Can you work these out from the drawing? Everything is in mm from the part's minimum corner. Round coordinates to 2 decimals unless told otherwise and drop trailing zeros. Write each loop counter-clockwise with the first axis right and the second up, starting at its lowest first coordinate (ties: lowest second). Pieces come first, ordered by that corner, then holes. Notation, with made-up numbers: (3.25, 14.25) - (49.25, 14.25) arc R30 ccw to (49.25, 36.25) - close; hole circle Ø6 at (-12, 71.25). An arc over 180 degrees is marked (long way). One line per item, written item: value. Start each with the question number.
(1) I want a section at C-C on y = 21. List the corners of the cut face in (x, z) for me.
(2) I want a section at D-D on z = 45. List the corners of the cut face in (x, y) for me.
(3) If I drill on L1, parallel to Y at x = 17.5, z = 50.5; L2, parallel to Y at x = 87.5, z = 52; L3, parallel to X at y = 11, z = 13.5, over which ranges is the centre line in solid material (lowest first)? Write a range as from..to.
(4) I want a section at B-B on x = 9. List the corners of the cut face in (y, z) for me.
(5) I want a section at A-A on z = 38.5. List the corners of the cut face in (x, y) for me.
(6) I'm going to push flat-ended pins straight in: pin 1 Ø6 at (x, y) = (85, 24) entering from +Z; pin 2 Ø6 at (x, z) = (51, 41) entering from -Y; pin 3 Ø1.5 at (x, z) = (36.5, 49.5) entering from -Y (3 decimals); pin 4 Ø12 at (x, z) = (12, 11.5) entering from -Y. Where does each tip first touch, or does it pass through?
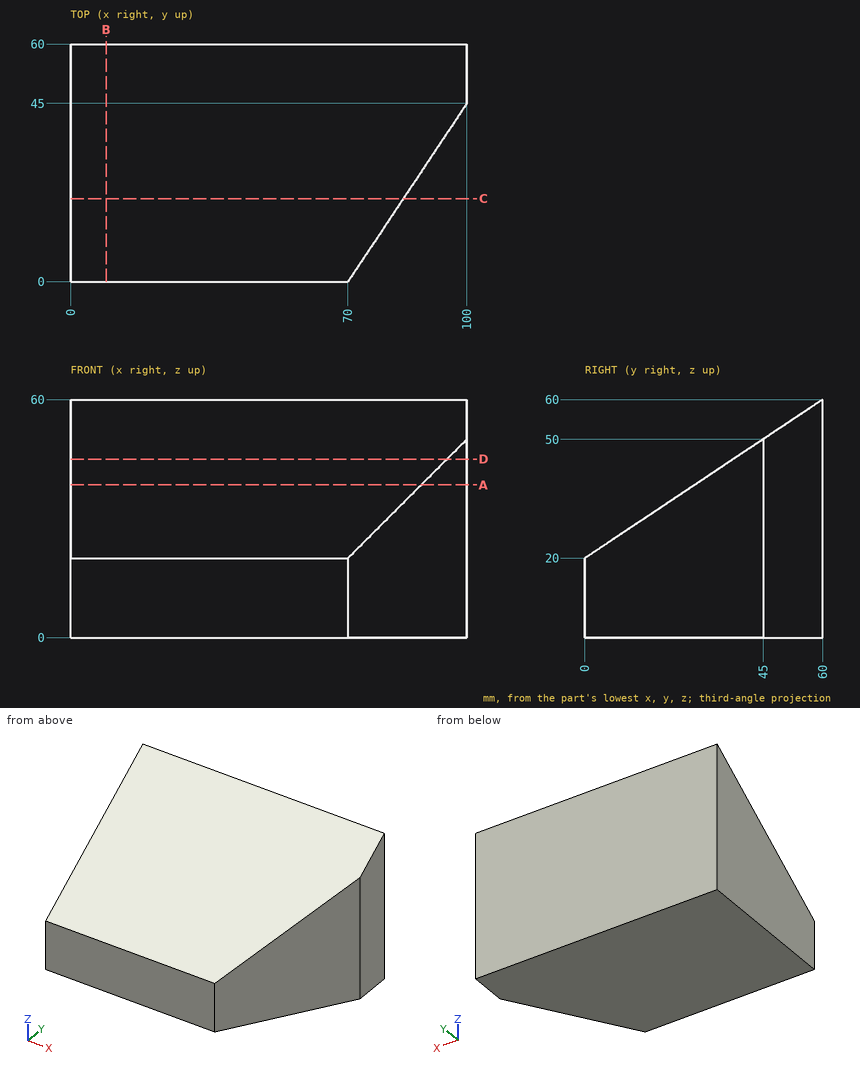
Established:
1. outline: (0, 0) - (84, 0) - (84, 34) - (0, 34) - close
2. outline: (0, 37.5) - (95, 37.5) - (100, 45) - (100, 60) - (0, 60) - close
3. L1: 45.75..60
3. L2: 48..60
3. L3: 0..77.33
4. outline: (0, 0) - (60, 0) - (60, 60) - (0, 20) - close
5. outline: (0, 27.75) - (88.5, 27.75) - (100, 45) - (100, 60) - (0, 60) - close
6. pin 1: z = 38
6. pin 2: y = 27
6. pin 3: y = 43.125
6. pin 4: y = 0
